Can you work these out from the model? Positions are in its coordinate system, mm. A direction names the side the tool comes from. Give positions to 0.01 mm unless a question says otherwise; leave off trailing zeros. Loops run counter-clockwise (first coordinate to the right, second up) from the corner with the lowest first, then second, coordinate; pieces in that order, holes last. Notation, with made-up numbers: M 80,-26 L 114,-26 A22 cw 114,-9 Z; hole C 35.5,18 d2. An arc over 180 degrees is marked long. One line per item, written item: value. Start each with the question number.
from build123d import *

# Parameters (mm, degrees)
BOSS_EXTRUDE1_DEPTH     = 10
BOSS_EXTRUDE2_DEPTH     = 27.5
BOSS_EXTRUDE3_DEPTH     = 10
CUT_EXTRUDE1_DEPTH      = 146.564029734
CUT_EXTRUDE1_DEPTH_BACK = 146.564029734


with BuildPart() as part:
    # Sketch1 → Boss-Extrude1 (new body)
    with BuildSketch(Plane(origin=(0, 0, 0), x_dir=(1, 0, 0), z_dir=(0, 1, 0))):
        with BuildLine():
            Line((-30, 104.285653561), (-30, 38.155653561))
            ThreePointArc((-30, 38.155653561), (0, 8.155653561), (30, 38.155653561))
            Line((30, 38.155653561), (30, 104.285653561))
            ThreePointArc((30, 104.285653561), (0, 134.285653561), (-30, 104.285653561))
        make_face()
    extrude(amount=BOSS_EXTRUDE1_DEPTH)

    # Sketch2 → Boss-Extrude2 (add)
    with BuildSketch(Plane(origin=(0, 10, 0), x_dir=(1, 0, 0), z_dir=(0, 1, 0))):
        with BuildLine():
            Line((-25, 104.285653561), (-25, 38.155653561))
            ThreePointArc((-25, 38.155653561), (0, 13.155653561), (25, 38.155653561))
            Line((25, 38.155653561), (25, 104.285653561))
            ThreePointArc((25, 104.285653561), (0, 129.285653561), (-25, 104.285653561))
        make_face()
    extrude(amount=BOSS_EXTRUDE2_DEPTH)

    # Sketch3 → Boss-Extrude3 (add)
    with BuildSketch(Plane(origin=(0, 37.5, 0), x_dir=(1, 0, 0), z_dir=(0, 1, 0))):
        with BuildLine():
            Line((-30, 104.285653561), (-30, 38.155653561))
            ThreePointArc((-30, 38.155653561), (0, 8.155653561), (30, 38.155653561))
            Line((30, 38.155653561), (30, 104.285653561))
            ThreePointArc((30, 104.285653561), (0, 134.285653561), (-30, 104.285653561))
        make_face()
    extrude(amount=BOSS_EXTRUDE3_DEPTH)

    # Sketch4 → Cut-Extrude1 (cut, two sides: drawn at the far end of the back side and taken through both)
    with BuildSketch(Plane(origin=(0, 47.5, 0), x_dir=(1, 0, 0), z_dir=(0, 1, 0)).offset(-CUT_EXTRUDE1_DEPTH_BACK)):
        with BuildLine():
            Line((-17.2, 99.020653561), (-17.2, 43.420653561))
            ThreePointArc((-17.2, 43.420653561), (0, 26.220653561), (17.2, 43.420653561))
            Line((17.2, 43.420653561), (17.2, 99.020653561))
            ThreePointArc((17.2, 99.020653561), (0, 116.220653561), (-17.2, 99.020653561))
        make_face()
    extrude(amount=CUT_EXTRUDE1_DEPTH + CUT_EXTRUDE1_DEPTH_BACK, mode=Mode.SUBTRACT)


solid = part.part
Q1. For P1, Ø14, axis at y = 26, z = -55.5, coming from the +X side; P2, Ø12, axis at x = -3.5, y = 24, coming from the +Z side; P3, Ø6, axis at x = -15.5, y = 22.5, coming from the +Z side (3 decimals), each with a flat end and sliding along its axis, tell me the tip position at first contact or that it passes through.
Q2. If we section it at A-A, the plane x = 0: Write out the boundary of the cut face in (y, z).
Q3. Which directions (+Z, -Z, +X, -X, +Y, -Y) give clear straight access to the entire face, cutting with the end or side of a thin tool? Please do faces 1 (the face through (0.55, 23.56, -129.28)), 2 (the face through (-25, 24, -72)), 3 (the face through (-27, 10, -72)), 4 (the face through (0.378, 23.418, -116.216)).
Q4. If we section it at C-C, the plane z = -97.5: Write out the boundary of the cut face in (x, y), plus the area to 3 significant figures.
Q5. If we section it at B-B, the plane y = 18: Write out the boundary of the cut face in (x, z), plus the area to 3 significant figures.
Q6. If we section it at D-D, the plane y = 43: Write out the boundary of the cut face in (x, z), plus the area to 3 significant figures.
Q7. I need wall thicknesses on line 1 along X through (y, z) = (36.5, -79.5); line 2 along Y through (x, z) = (27.5, -30.5); line 3 along X through (y, z) = (4.5, -77.5). Which ranges of each line are inside material? Lowest first, please.
Q8. If we mould it in two halves opening along Z, with no side actions, what happens to faces 5 (the face through (20, 47.5, -72)), 6 (the face through (-0.55, 23.56, -13.16)), 7 (the face through (-17.2, 23, -72))? For each: released by +Z, released by -Z, zero draft, split by the parting line, or undercut.
Response:
1. P1: x = 25
1. P2: z = -13.16
1. P3: z = -16.505
2. outline: M 0,-134.29 L 10,-134.29 L 10,-129.29 L 37.5,-129.29 L 37.5,-134.29 L 47.5,-134.29 L 47.5,-116.22 L 0,-116.22 Z; M 0,-26.22 L 47.5,-26.22 L 47.5,-8.16 L 37.5,-8.16 L 37.5,-13.16 L 10,-13.16 L 10,-8.16 L 0,-8.16 Z
3. face 1: -Z
3. face 2: +Z, -Z, -X
3. face 3: none
3. face 4: +Y, -Y
4. outline: M -30,0 L -17.2,0 L -17.2,47.5 L -30,47.5 L -30,37.5 L -25,37.5 L -25,10 L -30,10 Z; M 17.2,0 L 30,0 L 30,10 L 25,10 L 25,37.5 L 30,37.5 L 30,47.5 L 17.2,47.5 Z
4. area: 941 mm^2
5. outline: M -25,-104.29 A25 ccw 25,-104.29 L 25,-38.16 A25 ccw -25,-38.16 Z; hole M -17.2,-99.02 A17.2 ccw 17.2,-99.02 L 17.2,-43.42 A17.2 ccw -17.2,-43.42 Z
5. area: 2,430 mm^2
6. outline: M -30,-104.29 A30 ccw 30,-104.29 L 30,-38.16 A30 ccw -30,-38.16 Z; hole M -17.2,-99.02 A17.2 ccw 17.2,-99.02 L 17.2,-43.42 A17.2 ccw -17.2,-43.42 Z
6. area: 3,950 mm^2
7. line 1: -25 to -17.2, 17.2 to 25
7. line 2: 0 to 10, 37.5 to 47.5
7. line 3: -30 to -17.2, 17.2 to 30
8. face 5: zero draft
8. face 6: released by +Z
8. face 7: undercut
